Verification items for the finished model (mm, model axes). A direction names the side the tool comes from. Round coordinates to 2 decimals unless told otherwise and drop trailing zeros. Order: outer loops, then holes, each group sorted by start corner. A loop starts at its lowest first (then second) coordinate and runs counter-clockwise, first axis right, second up. Notation, with made-up numbers: (73.25, 25) -> (130.25, 25) arc R20 cw to (130.25, 42) -> close; hole circle Ø2 at (5, 26). An arc over 180 degrees is marked (long way). Answer in a Markdown table with one row per item. Add a question column.
```python
from build123d import *

# Parameters (mm, degrees)
SKETCH1_W           = 22.606
SKETCH1_H           = 12.446
BOSS_EXTRUDE1_DEPTH = 18.415
BOSS_EXTRUDE2_DEPTH = 2.54
SKETCH3_W           = 22.606
SKETCH3_H           = 12.446
BOSS_EXTRUDE3_DEPTH = 1.651
BOSS_EXTRUDE4_DEPTH = 5.842
SKETCH5_R           = 2.413
BOSS_EXTRUDE5_DEPTH = 4.318


with BuildPart() as part:
    # Sketch1 → Boss-Extrude1 (new body)
    with BuildSketch(Plane(origin=(0, 0, 0), x_dir=(1, 0, 0), z_dir=(0, 1, 0))):
        Rectangle(SKETCH1_W, SKETCH1_H)
    extrude(amount=BOSS_EXTRUDE1_DEPTH)

    # Sketch2 → Boss-Extrude2 (add)
    with BuildSketch(Plane(origin=(0, 18.415, 0), x_dir=(1, 0, 0), z_dir=(0, 1, 0))):
        with BuildLine():
            Line((15.875, -6.223), (-15.875, -6.223))
            Line((-15.875, -6.223), (-15.875, -0.889))
            Line((-15.875, -0.889), (-14.605, -0.889))
            ThreePointArc((-14.605, -0.889), (-12.74357951, 0), (-14.605, 0.889))
            Line((-14.605, 0.889), (-15.875, 0.889))
            Line((-15.875, 0.889), (-15.875, 6.223))
            Line((-15.875, 6.223), (15.875, 6.223))
            Line((15.875, 6.223), (15.875, 0.889))
            Line((15.875, 0.889), (14.605, 0.889))
            ThreePointArc((14.605, 0.889), (12.74357951, 0), (14.605, -0.889))
            Line((14.605, -0.889), (15.875, -0.889))
            Line((15.875, -0.889), (15.875, -6.223))
        make_face()
    extrude(amount=BOSS_EXTRUDE2_DEPTH)

    # Sketch3 → Boss-Extrude3 (add)
    with BuildSketch(Plane(origin=(0, 20.955, 0), x_dir=(1, 0, 0), z_dir=(0, 1, 0))):
        Rectangle(SKETCH3_W, SKETCH3_H)
    extrude(amount=BOSS_EXTRUDE3_DEPTH)

    # Sketch4 → Boss-Extrude4 (add)
    with BuildSketch(Plane(origin=(0, 22.606, 0), x_dir=(1, 0, 0), z_dir=(0, 1, 0))):
        with BuildLine():
            ThreePointArc((0.656127614, -2.413), (-6.310814133, -6.100067669), (-11.303, 0))
            ThreePointArc((-11.303, 0), (-6.310814133, 6.100067669), (0.656127614, 2.413))
            Line((0.656127614, 2.413), (1.143, 2.413))
            ThreePointArc((1.143, 2.413), (3.556, 0), (1.143, -2.413))
            Line((1.143, -2.413), (0.656127614, -2.413))
        make_face()
    extrude(amount=BOSS_EXTRUDE4_DEPTH)

    # Sketch5 → Boss-Extrude5 (add)
    with BuildSketch(Plane(origin=(0, 28.448, 0), x_dir=(1, 0, 0), z_dir=(0, 1, 0))):
        with Locations((-5.08, 0)):
            Circle(SKETCH5_R)
    extrude(amount=BOSS_EXTRUDE5_DEPTH)


solid = part.part
```
1) Thickness scan on L1, parallel to X at y = 18, z = -5; L2, parallel to Y at x = 8.5, z = 3; L3, parallel to X at y = 19.7, z = 0. Record the ranges inside material, lowest first. Write a range as [from, to].
2) Cross-section at B-B, the plane z = -4.25. Record the boundary of the cut face in (x, y) (3 decimals).
3) Cross-section at C-C, the plane x = 6. Record the boundary of the cut face in (y, z).
4) Cross-section at D-D, the plane y = 30. Record the boundary of the cut face in (x, z), and give its area (3 significant figures).
5) Depth check by flat-ended pin: P1, Ø3, axis at x = -8.5, z = -3.5, coming from the +Y side; P2, Ø0.8, axis at y = 21.5, z = -1.5, coming from the +X side; P3, Ø3.5, axis at x = -14.5, z = 2, coming from the -Y side (3 decimals). Enter the tip coordinate at first touch or a pass-through.
6) Draft check along X on faces 5 (the face through (-12.744, 19.667, 0.036)), 6 (the face through (-10, 22.606, -5)), 7 (the face through (-11.303, 22, 0)). Enter one of: +X half, -X half, draft (parallel to the pull), parting line (faces both ways), or undercut.
7) Tool access check on faces 1 (the face through (-15, 20, 0.889)), 2 (the face through (-11.303, 9, 0)), 3 (the face through (3.555, 25.486, -0.053)), 4 (the face through (15, 20, 0.889)). Record the directions out of +Z, -Z, +X, -X, +Y, -Y that give a thin tool (end or side, any length) a straight path to the whole face; none if there is none.
8) Cross-section at A-A, the plane x = 13.5. Record the boundary of the cut face in (y, z) (3 decimals), and give its area (3 significant figures).
Results below:
| question | item | result |
|---|---|---|
| 1 | L1 | [-11.3, 11.3] |
| 1 | L2 | [0, 22.61] |
| 1 | L3 | [-12.74, 12.74] |
| 2 | outline | (-15.875, 18.415) -> (-11.303, 18.415) -> (-11.303, 0) -> (11.303, 0) -> (11.303, 18.415) -> (15.875, 18.415) -> (15.875, 20.955) -> (11.303, 20.955) -> (11.303, 22.606) -> (-0.534, 22.606) -> (-0.534, 28.448) -> (-9.626, 28.448) -> (-9.626, 22.606) -> (-11.303, 22.606) -> (-11.303, 20.955) -> (-15.875, 20.955) -> close |
| 3 | outline | (0, -6.22) -> (22.61, -6.22) -> (22.61, 6.22) -> (0, 6.22) -> close |
| 4 | outline | circle Ø4.83 at (-5.08, 0) |
| 4 | area | 18.3 mm² |
| 5 | P1 | y = 28.45 |
| 5 | P2 | x = 11.3 |
| 5 | P3 | y = 18.415 |
| 6 | face 5 | undercut |
| 6 | face 6 | draft |
| 6 | face 7 | -X half |
| 7 | face 1 | -X, +Y, -Y |
| 7 | face 2 | +Z, -Z, -X, -Y |
| 7 | face 3 | +X, +Y |
| 7 | face 4 | +X, +Y, -Y |
| 8 | outline | (18.415, -6.223) -> (20.955, -6.223) -> (20.955, -1.076) -> (18.415, -1.076) -> close; (18.415, 1.076) -> (20.955, 1.076) -> (20.955, 6.223) -> (18.415, 6.223) -> close |
| 8 | area | 26.1 mm² |
